Check sheet for the modelled part. Datum: model origin and axes. Units: mm. Round coordinates to 2 decimals unless told otherwise and drop trailing zeros. Loops run counter-clockwise (first coordinate to the right, second up) from the corner with the lowest first, then second, coordinate; pieces in that order, holes last. Notation, with made-up numbers: (19, -11) - (56, -11) arc R19 ccw to (56, 23) - close; hole circle Ø6 at (46.25, -26). An arc over 180 degrees is marked (long way). Return JSON: item names as keys, results as strings.
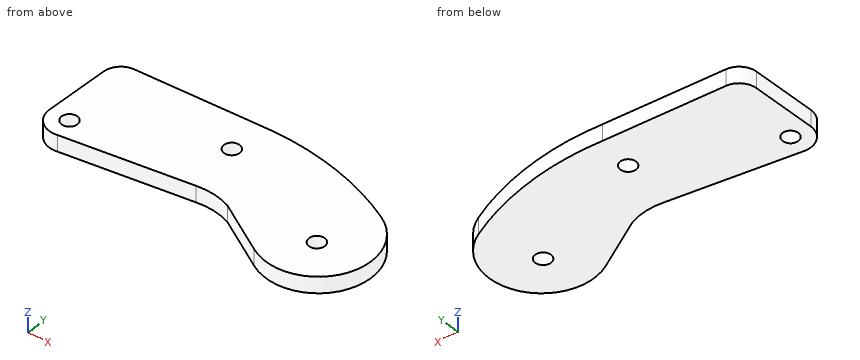
from build123d import *

# Parameters (mm, degrees)
SKETCH1_R           = 3
BOSS_EXTRUDE1_DEPTH = 6.2


with BuildPart() as part:
    # Sketch1 → Boss-Extrude1 (new body)
    with BuildSketch(Plane.XY):
        with BuildLine():
            Line((-44, -26.8), (2.7, -20.15))
            ThreePointArc((2.7, -20.15), (9.249876076, -19.98611928), (15.6, -21.599705241))
            Line((15.6, -21.599705241), (34.768435899, -32.920104396))
            ThreePointArc((34.768435899, -32.920104396), (62.542861937, -25.448265408), (54.469609674, 2.157344845))
            ThreePointArc((54.469609674, 2.157344845), (27.320189876, 11.997539893), (-1.5, 13.818827736))
            Line((-1.5, 13.818827736), (-45.886645473, 11.5))
            ThreePointArc((-45.886645473, 11.5), (-50.294249478, 9.530490598), (-52.238519213, 5.111694886))
            Line((-52.238519213, 5.111694886), (-53.366350091, -19.138305114))
            ThreePointArc((-53.366350091, -19.138305114), (-50.517454676, -25.21154219), (-44, -26.8))
        make_face()
        with Locations(Location((47, -18.8, 0), (0, 0, 180))):
            Circle(SKETCH1_R, mode=Mode.SUBTRACT)
        with Locations(Location((-45.6, -19.2, 0), (0, 0, 180))):
            Circle(SKETCH1_R, mode=Mode.SUBTRACT)
        with Locations(Location((0, 0, 0), (0, 0, 180))):
            Circle(SKETCH1_R, mode=Mode.SUBTRACT)
    extrude(amount=BOSS_EXTRUDE1_DEPTH)


solid = part.part
Q1. Scan lines: probe 1 along Y at (x, z) = (-45.6, 1.5); probe 2 along X at (y, z) = (-18.8, 2.25); probe 3 along X at (y, z) = (-19.2, 3.25). Record each from-to range of solid material in increasing order. Write a range as [from, to].
Answer key:
{"probe 1": "y = [-26.97, -22.2], [-16.2, 11.51]", "probe 2": "x = [-53.35, -48.57], [-42.63, 44], [50, 64.86]", "probe 3": "x = [-53.37, -48.6], [-42.6, 44.03], [49.97, 64.79]"}
Q2. Sectioned sample at A-A (z = 1.25). Enter the section's corners in (x, y).
Answer key:
{"outline": "(-53.37, -19.14) arc R7.77 ccw to (-44, -26.8) - (2.7, -20.15) arc R24 cw to (15.6, -21.6) - (34.77, -32.92) arc R20.12 ccw (long way) to (54.47, 2.16) arc R101.81 ccw to (-1.5, 13.82) - (-45.89, 11.5) arc R6.71 ccw to (-52.24, 5.11) - close; hole circle Ø6 at (-45.6, -19.2); hole circle Ø6 at (0, 0); hole circle Ø6 at (47, -18.8)"}
Q3. Depth check by flat-ended pin: P1, Ø2, axis at y = -22.5, z = 2, coming from the +X side; P2, Ø12, axis at x = -15.5, y = -25.5, coming from the -Z side; P3, Ø1.5, axis at x = 13, z = 3.5, coming from the +Y side; P4, Ø1.5, axis at y = -20.5, z = 2, coming from the +X side. Enter the tip coordinate at first touch or a pass-through.
Answer key:
{"P1": "stops at x = 64.23", "P2": "stops at z = 0", "P3": "stops at y = 13.98", "P4": "stops at x = 64.69"}
Q4. Sectioned sample at C-C (y = 0). Enter the section's corners in (x, z).
Answer key:
{"outline": "(-52.48, 0) - (-3, 0) - (-3, 6.2) - (-52.48, 6.2) - close; (3, 0) - (57.71, 0) - (57.71, 6.2) - (3, 6.2) - close"}
Q5. Sectioned sample at D-D (x = -34.5). Enter the section's corners in (y, z).
Answer key:
{"outline": "(-25.45, 0) - (12.09, 0) - (12.09, 6.2) - (-25.45, 6.2) - close"}
Q6. Sectioned sample at B-B (x = 0). Enter the section's corners in (y, z).
Answer key:
{"outline": "(-20.53, 0) - (-3, 0) - (-3, 6.2) - (-20.53, 6.2) - close; (3, 0) - (13.93, 0) - (13.93, 6.2) - (3, 6.2) - close"}
